from build123d import *

# Parameters (mm, degrees)
F0_W     = 406.4
F0_H     = 38.1
F1_DEPTH = 9.525
F2_W     = 254
F2_H     = 9.779
F3_DEPTH = 9.526
F4_R     = 6.35
F5_W     = 406.4
F5_H     = 6.35
F6_DEPTH = 1.778
F7_R     = 4.507099
F7_R_2   = 4.388412
F8_DEPTH = 9.526
F9_SIZE  = 0.762


with BuildPart() as f1:
    # F0 (on Front) → F1 (new body)
    with BuildSketch(Plane.XZ):
        Rectangle(F0_W, F0_H)
    extrude(amount=F1_DEPTH)

    # F2 (on face) → F3 (cut, through all)
    with BuildSketch(Plane.XZ.offset(9.525)):
        with Locations((0, -14.1605)):
            Rectangle(F2_W, F2_H)
    extrude(amount=-F3_DEPTH, mode=Mode.SUBTRACT)

    # F4
    f4_edges = [f1.edges().sort_by_distance(p)[0] for p in [
        (-127, -4.7625, -9.271),
        (127, -4.7625, -9.271),
    ]]
    fillet(f4_edges, radius=F4_R)

    # F5 (on face) → F6 (cut)
    with BuildSketch(Plane.XZ.offset(9.525)):
        with Locations((0, 15.875)):
            Rectangle(F5_W, F5_H)
    extrude(amount=-F6_DEPTH, mode=Mode.SUBTRACT)

    # F7 (on face) → F8 (cut, through all)
    with BuildSketch(Plane.XZ.offset(9.525)):
        with Locations((139.7, -9.525)):
            Circle(F7_R)
        with Locations((177.8, -9.525)):
            Circle(F7_R_2)
        with Locations((-177.8, -9.525)):
            Circle(F7_R_2)
        with Locations((-139.7, -9.525)):
            Circle(F7_R)
    extrude(amount=-F8_DEPTH, mode=Mode.SUBTRACT)

    # F9
    f9_edges = [f1.edges().sort_by_distance(p)[0] for p in [
        (-182.188412, -9.525, -9.525),
        (-144.207099, -9.525, -9.525),
        (135.192901, -9.525, -9.525),
        (173.411588, -9.525, -9.525),
        (173.411588, 0, -9.525),
        (135.192901, 0, -9.525),
        (-144.207099, 0, -9.525),
        (-182.188412, 0, -9.525),
    ]]
    chamfer(f9_edges, length=F9_SIZE)


solid = f1.part
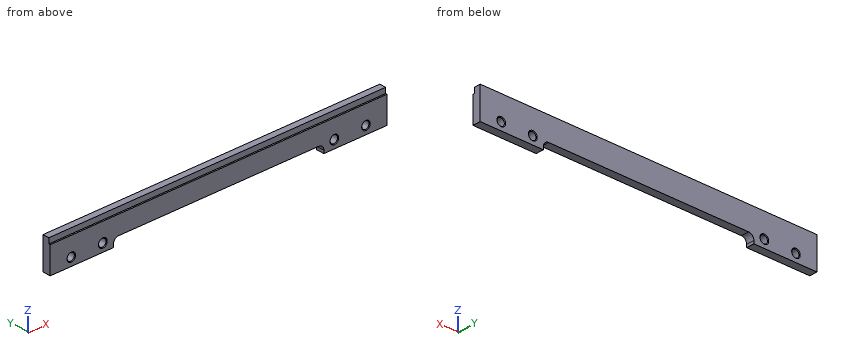
Build history of the part. All positions in model axes, mm. Give positions to 0.01 mm unless a question says otherwise; leave off trailing zeros. Order: outer loops, then holes, each group sorted by start corner. A loop starts at its lowest first (then second) coordinate and runs counter-clockwise, first axis right, second up. Notation, with made-up numbers: M -25,45 L -7,45 A36 ccw -7,81 Z; hole C 17,47.25 d6. An arc over 180 degrees is marked long. Use one line per item in the form item = value.
Q1. Slice it at D-D, the plane x = 163. Write the cut outline in (y, z) (3 decimals).
Conclusion:
outline = M -9.525,-19.05 L 0,-19.05 L 0,19.05 L -7.747,19.05 L -7.747,12.7 L -9.525,12.7 Z
Q2. Wall check: probe 1 along X at (y, z) = (-6, -12); probe 2 along X at (y, z) = (-8, -13.5); probe 3 along Z at (x, y) = (-139.7, -3). Give the ranges that are in metal, low to high.
Conclusion:
probe_1 = -203.2 to -181.42, -174.18 to -143.47, -135.93 to -125.87, 125.87 to 135.93, 143.47 to 174.18, 181.42 to 203.2
probe_2 = -203.2 to -179.66, -175.94 to -141.82, -137.58 to -126.64, 126.64 to 137.58, 141.82 to 175.94, 179.66 to 203.2
probe_3 = -19.05 to -14.03, -5.02 to 19.05
Q3. Slice it at C-C, the plane x = 20. Write the cut outline in (y, z) (3 decimals), and give its area (3 significant figures).
Conclusion:
outline = M -9.525,-9.271 L 0,-9.271 L 0,19.05 L -7.747,19.05 L -7.747,12.7 L -9.525,12.7 Z
area = 258 mm2
Q4. Pin check, flat tips, straight feed: P1, Ø4, axis at x = 86.5, y = -4, coming from the -Z side; P2, Ø0.5, axis at x = 41, y = -9, coming from the +Z side. Stop position of each tip, or through.
Conclusion:
P1 = -9.27
P2 = 12.7
Q5. Slice it at A-A, the plane x = -139.7. Write the cut outline in (y, z) (3 decimals), and give its area (3 significant figures).
Conclusion:
outline = M -9.525,-19.05 L 0,-19.05 L 0,-14.794 L -0.762,-14.032 L -8.763,-14.032 L -9.525,-14.794 Z; M -9.525,-4.256 L -8.763,-5.018 L -0.762,-5.018 L 0,-4.256 L 0,19.05 L -7.747,19.05 L -7.747,12.7 L -9.525,12.7 Z
area = 265 mm2
Q6. Slice it at B-B, the plane y = -4.5. Write the cut outline in (x, z) (3 decimals).
Conclusion:
outline = M -203.2,-19.05 L -127,-19.05 L -127,-15.621 A6.35 cw -120.65,-9.271 L 120.65,-9.271 A6.35 cw 127,-15.621 L 127,-19.05 L 203.2,-19.05 L 203.2,19.05 L -203.2,19.05 Z; hole C -177.8,-9.525 d8.777; hole C -139.7,-9.525 d9.014; hole C 139.7,-9.525 d9.014; hole C 177.8,-9.525 d8.777
